from build123d import *

# Parameters (mm, degrees)
SKETCH27_W                    = 107.95
SKETCH27_H                    = 152.4
BOSS_EXTRUDE4_DEPTH           = 38.1
CUT_EXTRUDE5_DEPTH            = 101.853114107
CUT_EXTRUDE5_DEPTH_BACK       = 101.853114107
CUT_EXTRUDE6_DEPTH            = 101.853114107
CUT_EXTRUDE6_DEPTH_BACK       = 101.853114107
SKETCH30_OUTSIDE_W            = 118.542
SKETCH30_OUTSIDE_H            = 194.742
F_3_8_CLEARANCE_HOLE4_D       = 10.31748
CUT_EXTRUDE8_REACH            = 139.518
SKETCH49_W                    = 22.54
SKETCH49_H                    = 42.54
M2_CLEARANCE_HOLE2_AT_2_COUNT = 2
M2_CLEARANCE_HOLE2_AT_2_PITCH = 10
M2_CLEARANCE_HOLE2_AT_3_COUNT = 2
M2_CLEARANCE_HOLE2_AT_3_PITCH = 49.030602689
M2_CLEARANCE_HOLE2_AT_4_COUNT = 2
M2_CLEARANCE_HOLE2_AT_4_PITCH = 48
F_1_4_CLEARANCE_HOLE1_D       = 7.14248
SKETCH53_W                    = 11.4935
SKETCH53_H                    = 11.4935
CUT_EXTRUDE9_DEPTH            = 6.8326
F_3_8_CLEARANCE_HOLE5_D       = 13.97


with BuildPart() as part:
    # Sketch27 → Boss-Extrude4 (new, symmetric)
    with BuildSketch(Plane.XY):
        Rectangle(SKETCH27_W, SKETCH27_H)
    extrude(amount=BOSS_EXTRUDE4_DEPTH, both=True)

    # Sketch28 → Cut-Extrude5 (cut, two sides: drawn at the far end of the back side and taken through both)
    with BuildSketch(Plane.XY.offset(-CUT_EXTRUDE5_DEPTH_BACK)):
        Polygon((-34.925, 439.068077332), (-34.925, 76.2), (-34.925, -57.15), (34.925, -57.15), (34.925, 76.2), (34.925, 439.068077332), (34.925, 1164.804231996), (-34.925, 1164.804231996), align=None)
    extrude(amount=CUT_EXTRUDE5_DEPTH + CUT_EXTRUDE5_DEPTH_BACK, mode=Mode.SUBTRACT)

    # Sketch30 outside → Cut-Extrude6 (cut, two sides: drawn at the far end of the back side and taken through both)
    with BuildSketch(Plane(origin=(0, 0, 0), x_dir=(0, 0, -1), z_dir=(1, 0, 0)).offset(-CUT_EXTRUDE6_DEPTH_BACK)):
        Rectangle(SKETCH30_OUTSIDE_W, SKETCH30_OUTSIDE_H)
        Polygon((-38.1, 50.8), (-38.1, -76.2), (38.1, -76.2), (38.1, 50.8), (12.7, 76.2), (-12.7, 76.2), align=None, mode=Mode.SUBTRACT)
    extrude(amount=CUT_EXTRUDE6_DEPTH + CUT_EXTRUDE6_DEPTH_BACK, mode=Mode.SUBTRACT)

    # 3/8 Clearance Hole4 (through all)
    with Locations(Plane.ZY.offset(53.975)):
        with Locations((0, 38.1)):
            Hole(F_3_8_CLEARANCE_HOLE4_D / 2)

    # Sketch49 → Cut-Extrude8 (cut, up to next)
    with BuildSketch(Plane(origin=(53.975, 0, 0), x_dir=(0, 0, -1), z_dir=(1, 0, 0)), mode=Mode.PRIVATE) as cut_extrude8_sk1:
        with Locations((0, -24.816666667)):
            Rectangle(SKETCH49_W, SKETCH49_H)
    cut_extrude8_tool1 = extrude(cut_extrude8_sk1.sketch, amount=-CUT_EXTRUDE8_REACH, mode=Mode.PRIVATE) & part.part
    cut_extrude8 = cut_extrude8_tool1.solids().sort_by_distance((53.975, -24.816667, 0))[0]
    add(cut_extrude8, mode=Mode.SUBTRACT)

    # Sketch51 → M2 Clearance Hole2 (revolve, cut)
    with BuildSketch(Plane(origin=(53.975, -48.816666667, 5), x_dir=(0, 0, -1), z_dir=(0, 1, 0))):
        Polygon((0, 0), (0, 15.721028143), (1.2, 14.9999954), (1.2, 0), align=None)
    m2_clearance_hole2 = revolve(axis=Axis((60.325, -48.816666667, 5), (-1, 0, 0)), mode=Mode.SUBTRACT)

    # M2 Clearance Hole2 at 2: M2 Clearance Hole2 ×2
    with Locations(*[(0, 0, -i * M2_CLEARANCE_HOLE2_AT_2_PITCH) for i in range(1, M2_CLEARANCE_HOLE2_AT_2_COUNT)]):
        add(m2_clearance_hole2, mode=Mode.SUBTRACT)

    # M2 Clearance Hole2 at 3: M2 Clearance Hole2 ×2
    with Locations(*[Vector(0, 0.9789804197376051, -0.20395425411200102) * (i * M2_CLEARANCE_HOLE2_AT_3_PITCH) for i in range(1, M2_CLEARANCE_HOLE2_AT_3_COUNT)]):
        add(m2_clearance_hole2, mode=Mode.SUBTRACT)

    # M2 Clearance Hole2 at 4: M2 Clearance Hole2 ×2
    with Locations(*[(0, i * M2_CLEARANCE_HOLE2_AT_4_PITCH, 0) for i in range(1, M2_CLEARANCE_HOLE2_AT_4_COUNT)]):
        add(m2_clearance_hole2, mode=Mode.SUBTRACT)

    # Mirror2: Cut-Extrude8, M2 Clearance Hole2 across plane
    add(cut_extrude8.mirror(Plane(origin=(0, 0, 0), x_dir=(0, 0, 1), z_dir=(1, 0, 0))), mode=Mode.SUBTRACT)
    add(m2_clearance_hole2.mirror(Plane(origin=(0, 0, 0), x_dir=(0, 0, 1), z_dir=(1, 0, 0))), mode=Mode.SUBTRACT)

    # Mirror2 copy 1 sketch → Mirror2 copy 1 (revolve, cut)
    with BuildSketch(Plane(origin=(-53.975, -48.816666667, -5), x_dir=(0, 0, -1), z_dir=(0, 1, 0))):
        Polygon((0, 0), (0, -15.721028143), (1.2, -14.9999954), (1.2, 0), align=None)
    revolve(axis=Axis((-60.325, -48.816666667, -5), (-1, 0, 0)), mode=Mode.SUBTRACT)

    # Mirror2 copy 2 sketch → Mirror2 copy 2 (revolve, cut)
    with BuildSketch(Plane(origin=(-53.975, -0.816666667, -5), x_dir=(0, 0, -1), z_dir=(0, 1, 0))):
        Polygon((0, 0), (0, -15.721028143), (1.2, -14.9999954), (1.2, 0), align=None)
    revolve(axis=Axis((-60.325, -0.816666667, -5), (-1, 0, 0)), mode=Mode.SUBTRACT)

    # Mirror2 copy 3 sketch → Mirror2 copy 3 (revolve, cut)
    with BuildSketch(Plane(origin=(-53.975, -0.816666667, 5), x_dir=(0, 0, -1), z_dir=(0, 1, 0))):
        Polygon((0, 0), (0, -15.721028143), (1.2, -14.9999954), (1.2, 0), align=None)
    revolve(axis=Axis((-60.325, -0.816666667, 5), (-1, 0, 0)), mode=Mode.SUBTRACT)

    # 1/4 Clearance Hole1 (through all)
    with Locations(Plane(origin=(0, -57.15, 0), x_dir=(1, 0, 0), z_dir=(0, 1, 0))):
        with Locations((-15.875, 15.875)):
            f_1_4_clearance_hole1 = Hole(F_1_4_CLEARANCE_HOLE1_D / 2)

    # Sketch53 → Cut-Extrude9 (cut)
    with BuildSketch(Plane(origin=(0, -57.15, 0), x_dir=(1, 0, 0), z_dir=(0, 1, 0))):
        with Locations((-15.875, 15.875)):
            Rectangle(SKETCH53_W, SKETCH53_H)
    cut_extrude9 = extrude(amount=-CUT_EXTRUDE9_DEPTH, mode=Mode.SUBTRACT)

    # Sketch-Pattern1: 1/4 Clearance Hole1, Cut-Extrude9 at 3 more places
    with Locations((31.75, 0, 0), (31.75, 0, 31.75), (0, 0, 31.75)):
        add(f_1_4_clearance_hole1, mode=Mode.SUBTRACT)
        add(cut_extrude9, mode=Mode.SUBTRACT)

    # 3/8 Clearance Hole5 (through all)
    with Locations(Plane(origin=(0, -57.15, 0), x_dir=(1, 0, 0), z_dir=(0, 1, 0))):
        with Locations((0, 0)):
            Hole(F_3_8_CLEARANCE_HOLE5_D / 2)


with BuildPart() as body_2:
    # uxcell-FR6ZZ: read off the stored shape, not the designer's step
    # uxcell-FR6ZZ outline → uxcell-FR6ZZ (revolve)
    with BuildSketch(Plane.XY):
        Polygon((12.303125, 7.14375), (4.7625, 7.14375), (4.7625, -0.381), (11.1125, -0.381), (11.1125, 4.778375), (11.509375, 5.17525), (12.303125, 5.17525), align=None)
    revolve(axis=Axis((0, 0, 0), (0, 1, 0)))


with BuildPart() as body_2_1:
    # Body-Move/Copy2: read off the stored shape, not the designer's step
    # Body-Move/Copy2: moved
    add(body_2.part.moved(Location((0, -64.29375, 0))))


with BuildPart() as part_1:
    add(part.part)

    # Combine1: cut body 2
    add(body_2_1.part, mode=Mode.SUBTRACT)


solid = part_1.part
CAD build for the part. Positions are in the model's coordinates, mm. A direction names the side the tool comes from. Round coordinates to 2 decimals unless told otherwise and drop trailing zeros. Loops run counter-clockwise (first coordinate to the right, second up) from the corner with the lowest first, then second, coordinate; pieces in that order, holes last.
(1) Wall check: line 1 along Y through (x, z) = (49, 0); line 2 along X through (y, z) = (-36, -29.5) (3 decimals); line 3 along X through (y, z) = (-59, 19) (3 decimals). Give the ranges that are in metal, low to high.
(2) Cut at C-C (y = -40.5). Give the cut face in (x, z) (3 decimals).
(3) Cut at D-D (z = 28). Give the cut face in (x, y) (3 decimals).
(4) Cut at A-A (y = 62). Give the cut face in (x, z) (3 decimals).
(5) Two-plate mould, pull along X, no slides. Class faces 1 (the flat face through (35.2, -11.8, 38.1)), 2 (the flat face through (-16, -61, -10.128)), 3 (the flat face through (16, -61, -10.128)), 4 (the flat face through (53.975, -1, 1)): +X half, -X half, draft (parallel to the pull), parting line (faces both ways), or undercut.
(6) Drop flat-ended pins along their axis: pin 1 (1.9 mm diameter, centred on y = -48.82, z = 5, fed in from -X); pin 2 (2 mm diameter, centred on x = 17, z = -17, fed in from -Y); pin 3 (9.5 mm diameter, centred on x = 15.875, z = -15.875, fed in from +Y). Give the stop position or say it passes through.
(7) Which spindle directions (+Z, -Z, +X, -X, +Y, -Y) get a long thin tool onto all of the face, cutting with end or side? Do faces 5 (the flat face through (-45, -25, -11.27)), 6 (the flat face through (0.2, -64.675, 7.3)), 7 (the flat face through (-34.925, 10, -1)), 8 (the flat face through (44.3, 63.3, -25.6)). Say none if no direction does.
Findings below:
1. line 1: y = -76.2 to -46.09, -3.55 to 32.94, 43.26 to 76.2
1. line 2: x = -53.975 to -34.925, 34.925 to 53.975
1. line 3: x = -53.975 to -21.622, -10.128 to 10.128, 21.622 to 53.975
2. outline: (-53.975, -38.1) - (-34.925, -38.1) - (-34.925, -11.27) - (-53.975, -11.27) - close; (-53.975, 11.27) - (-34.925, 11.27) - (-34.925, 38.1) - (-53.975, 38.1) - close; (34.925, -38.1) - (53.975, -38.1) - (53.975, -11.27) - (34.925, -11.27) - close; (34.925, 11.27) - (53.975, 11.27) - (53.975, 38.1) - (34.925, 38.1) - close
3. outline: (-53.975, -76.2) - (53.975, -76.2) - (53.975, 60.9) - (34.925, 60.9) - (34.925, -57.15) - (-34.925, -57.15) - (-34.925, 60.9) - (-53.975, 60.9) - close
4. outline: (-53.975, -26.9) - (-34.925, -26.9) - (-34.925, 26.9) - (-53.975, 26.9) - close; (34.925, -26.9) - (53.975, -26.9) - (53.975, 26.9) - (34.925, 26.9) - close
5. face 1: draft
5. face 2: undercut
5. face 3: undercut
5. face 4: +X half
6. pin 1: stops at x = -38.83
6. pin 2: passes through
6. pin 3: stops at y = -63.98
7. face 5: +X, -X
7. face 6: +Y
7. face 7: +Z, -Z, +Y
7. face 8: -Z, +X, -X, +Y
